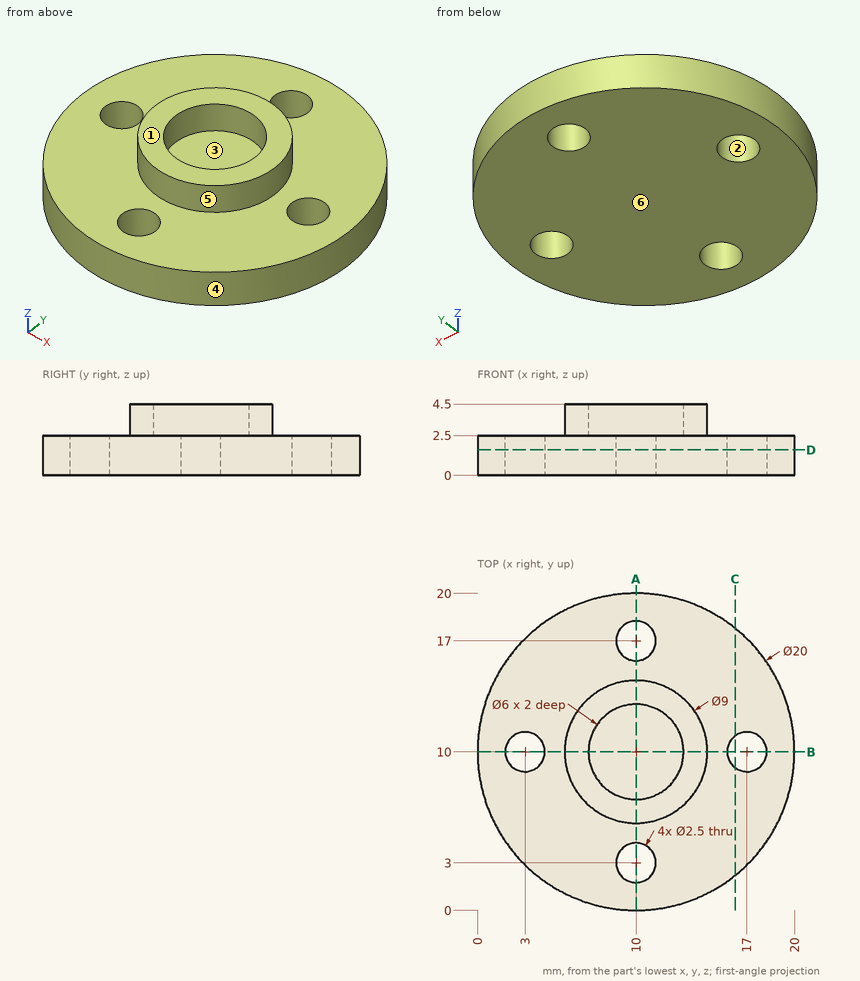
Study the drawing (mm; zero at the part's minimum x, y, z) and answer. A direction names the side the tool comes from. Round coordinates to 2 decimals unless told otherwise and drop trailing zeros. Write each loop counter-clockwise with the first axis right and the second up, starting at its lowest first coordinate (ties: lowest second). Pieces come first, ordered by that corner, then holes. Notation, with made-up numbers: (0, 33.5) - (11, 33.5) arc R26 ccw to (11, 51.5) - close; hole circle Ø11 at (-3, -17). An arc over 180 degrees is marked (long way). Return JSON: item names as keys, results as strings. Group by question number.
Q1. Each of these flat-tipped pins is pushed along its axis until it touches: pin 1 Ø3 at (x, y) = (17, 10) entering from +Z; pin 2 Ø1.5 at (x, z) = (3.5, 1.5) entering from +Y. Where does it stop, or does it pass through?
Q2. The part is cut by section A-A on x = 10. Write down the section's boundary in (y, z), then the cut area to 3 significant figures.
Q3. Find the intervals of material crossed by L1, parallel to Y at x = 10, z = 1.7; L2, parallel to Y at x = 9.25, z = 2.35; L3, parallel to Z at x = 2.75, y = 8, in increasing order.
Q4. The part is cut by section D-D on z = 1.6. Write down the section's boundary in (x, y).
Q5. The mould has two halves that part along X. Classify the marked faces 1, 2, 3 and 4: released by +X, released by -X, zero draft, split by the parting line, or undercut.
Q6. For the marked faces 5 and 6, determine the directions among +Z, -Z, +X, -X, +Y, -Y from which every point of the face is accessible in a straight line to the end or side of a thin tool.
Q7. The part is cut by section C-C on x = 16.25. Write down the section's boundary in (y, z).
Solved:
{
 "1": {"pin 1": "z = 2.5", "pin 2": "y = 18.18"},
 "2": {"outline": "(0, 0) - (1.75, 0) - (1.75, 2.5) - (0, 2.5) - close; (4.25, 0) - (15.75, 0) - (15.75, 2.5) - (14.5, 2.5) - (14.5, 4.5) - (13, 4.5) - (13, 2.5) - (7, 2.5) - (7, 4.5) - (5.5, 4.5) - (5.5, 2.5) - (4.25, 2.5) - close; (18.25, 0) - (20, 0) - (20, 2.5) - (18.25, 2.5) - close", "area": "43.5 mm²"},
 "3": {"L1": "0 to 1.75, 4.25 to 15.75, 18.25 to 20", "L2": "0.03 to 2, 4 to 16, 18 to 19.97", "L3": "0 to 2.5"},
 "4": {"outline": "circle Ø20 at (10, 10); hole circle Ø2.5 at (3, 10); hole circle Ø2.5 at (10, 3); hole circle Ø2.5 at (10, 17); hole circle Ø2.5 at (17, 10)"},
 "5": {"face 1": "zero draft", "face 2": "undercut", "face 3": "undercut", "face 4": "split by the parting line"},
 "6": {"face 5": "+Z", "face 6": "-Z, +X, -X, +Y, -Y"},
 "7": {"outline": "(2.19, 0) - (9, 0) - (9, 2.5) - (2.19, 2.5) - close; (11, 0) - (17.81, 0) - (17.81, 2.5) - (11, 2.5) - close"}
}
